Geometry: final body of the model. Coordinates: model frame, mm. A direction names the side the tool comes from. Give positions to 0.01 mm unless a question says otherwise; leave off trailing zeros. Write each loop counter-clockwise with the first axis right and the second up, starting at its lowest first coordinate (ties: lowest second). Pieces come first, ordered by that corner, then holes.
from build123d import *

# Parameters (mm, degrees)
BOSS_EXTRUDE1_DEPTH = 101.6
SKETCH5_R           = 11.1125
CUT_EXTRUDE1_DEPTH  = 125.434078933
SKETCH6_R           = 3.175
BOSS_EXTRUDE3_DEPTH = 25.4


with BuildPart() as part:
    # Sketch4 → Boss-Extrude1 (new body)
    with BuildSketch(Plane.XY):
        Polygon((0, 0), (0, 50.8), (50.8, 50.8), (50.8, 0), (38.1, 0), (38.1, 38.135977337), (12.7, 38.135977337), (12.7, 0), align=None)
    extrude(amount=BOSS_EXTRUDE1_DEPTH)

    # Sketch5 → Cut-Extrude1 (cut, through all)
    with BuildSketch(Plane.ZY):
        with Locations((13.716, 17.4625)):
            Circle(SKETCH5_R)
        with Locations((38.481, 17.4625)):
            Circle(SKETCH5_R)
        with Locations((63.246, 17.4625)):
            Circle(SKETCH5_R)
        with Locations((88.011, 17.4625)):
            Circle(SKETCH5_R)
    extrude(amount=-CUT_EXTRUDE1_DEPTH, mode=Mode.SUBTRACT)

    # Sketch6 → Boss-Extrude3 (add)
    with BuildSketch(Plane.XZ):
        with Locations(Location((6.35, 25.4, 0), (0, 0, 180))):
            Circle(SKETCH6_R)
        with Locations(Location((6.35, 76.2, 0), (0, 0, 180))):
            Circle(SKETCH6_R)
        with Locations(Location((44.45, 76.2, 0), (0, 0, 180))):
            Circle(SKETCH6_R)
        with Locations(Location((44.45, 25.4, 0), (0, 0, 180))):
            Circle(SKETCH6_R)
    extrude(amount=BOSS_EXTRUDE3_DEPTH)


solid = part.part
Q1. Ray query, line 1 along X through (y, z) = (30.5, 43.5); line 2 along X through (y, z) = (-16.5, 25); line 3 along Y through (x, z) = (12.5, 89.5). Return the intervals inside material, ascending.
Filled sheet:
line 1: x = 0 to 12.7, 38.1 to 50.8
line 2: x = 3.2 to 9.5, 41.3 to 47.6
line 3: y = 0 to 6.45, 28.47 to 50.8
Q2. Pull-direction query (Z, two-part tool) for faces 1 (the cylindrical face through (6.261, 17.951, 52.144)), 2 (the flat face through (26, 43, 101.6)), 3 (the flat face through (25, 50.8, 50)); classes: released by +Z, released by -Z, zero draft, split by the parting line, or undercut.
Filled sheet:
face 1: undercut
face 2: released by +Z
face 3: zero draft
Q3. Section A-A on x = 7. Output: boundary loops of the cut face in (y, z) (1 decimal).
Filled sheet:
outline: (-25.4, 22.3) - (0, 22.3) - (0, 0) - (50.8, 0) - (50.8, 101.6) - (0, 101.6) - (0, 79.3) - (-25.4, 79.3) - (-25.4, 73.1) - (0, 73.1) - (0, 28.5) - (-25.4, 28.5) - close; hole circle Ø22.2 at (17.5, 13.7); hole circle Ø22.2 at (17.5, 38.5); hole circle Ø22.2 at (17.5, 63.2); hole circle Ø22.2 at (17.5, 88)
Q4. Pin query (flat end, axial travel): P1, Ø20.5, axis at x = 28.5, z = 31.5, coming from the -Y side; P2, Ø13.5, axis at y = 17.46, z = 38.48, coming from the -X side; P3, Ø3, axis at x = 33.5, z = 67, coming from the -Y side. Return the tip coordinate at first contact, or that it passes through.
Filled sheet:
P1: stops at y = 0
P2: passes through
P3: stops at y = 38.14
Q5. Access query for faces 4 (the cylindrical face through (6.26, 17.95, 76.91)), 5 (the cylindrical face through (42.985, -12.522, 79.017)), 6 (the flat face through (38.1, 19, 50)). Directions: +Z, -Z, +X, -X, +Y, -Y. A direction counts if a zero-diameter tool reaches every point of the face in a straight line with its end or side. Return the directions, or none.
Filled sheet:
face 4: +X, -X
face 5: -Y
face 6: +Z, -Z, -Y
Q6. Section B-B on z = 93. Output: boundary loops of the cut face in (x, y), plus the area to 3 significant figures.
Filled sheet:
outline: (0, 0) - (12.7, 0) - (12.7, 7.53) - (0, 7.53) - close; (0, 27.39) - (12.7, 27.39) - (12.7, 38.14) - (38.1, 38.14) - (38.1, 27.39) - (50.8, 27.39) - (50.8, 50.8) - (0, 50.8) - close; (38.1, 0) - (50.8, 0) - (50.8, 7.53) - (38.1, 7.53) - close
area: 1,110 mm2
Q7. Section C-C on x = 16. Output: boundary loops of the cut face in (y, z), plus the area to 3 significant figures.
Filled sheet:
outline: (38.14, 0) - (50.8, 0) - (50.8, 101.6) - (38.14, 101.6) - close
area: 1,290 mm2
Q8. Section D-D on z = 8. Output: boundary loops of the cut face in (x, y), plus the area to 3 significant figures.
Filled sheet:
outline: (0, 0) - (12.7, 0) - (12.7, 7.93) - (0, 7.93) - close; (0, 26.99) - (12.7, 26.99) - (12.7, 38.14) - (38.1, 38.14) - (38.1, 26.99) - (50.8, 26.99) - (50.8, 50.8) - (0, 50.8) - close; (38.1, 0) - (50.8, 0) - (50.8, 7.93) - (38.1, 7.93) - close
area: 1,130 mm2
